Answer from the drawing. Dimensions are ordinates in mm from the lowest x, y and z of the part. Coordinates: 2 decimals unless noted, no trailing zeros. Loops run counter-clockwise (first coordinate to the right, second up) from the corner with the lowest first, then second, coordinate; pieces in that order, holes last. Notation, with made-up numbers: M 34,14 L 48,14 A22 ccw 48,53 Z; hole C -14,9 d11. An arc over 180 degrees is marked long. Answer as CSV lines item,"result". Start each with the question number.
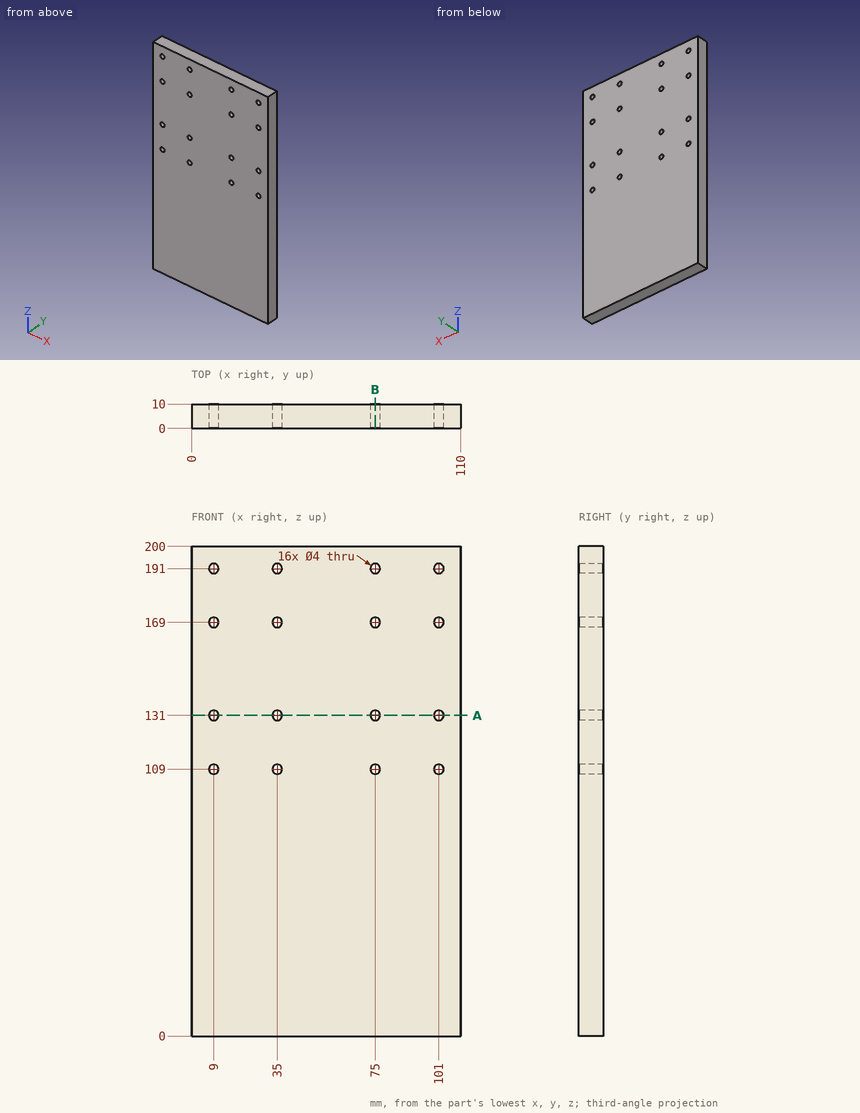
Item 1: Consider line 1 (Z direction, x = 75, y = 7.75); line 2 (X direction, y = 7.25, z = 169); line 3 (X direction, y = 8.25, z = 110.5). Determine where each line is inside the solid, lowest interval first.
Item 2: Section A-A on z = 131 is taken. Determine the outline of the cut face in (x, y).
Item 3: Section B-B on x = 75 is taken. Determine the outline of the cut face in (y, z).
Results are:
1,line 1,"0 to 107, 111 to 129, 133 to 167, 171 to 189, 193 to 200"
1,line 2,"0 to 7, 11 to 33, 37 to 73, 77 to 99, 103 to 110"
1,line 3,"0 to 7.68, 10.32 to 33.68, 36.32 to 73.68, 76.32 to 99.68, 102.32 to 110"
2,outline,"M 0,0 L 7,0 L 7,10 L 0,10 Z; M 11,0 L 33,0 L 33,10 L 11,10 Z; M 37,0 L 73,0 L 73,10 L 37,10 Z; M 77,0 L 99,0 L 99,10 L 77,10 Z; M 103,0 L 110,0 L 110,10 L 103,10 Z"
3,outline,"M 0,0 L 10,0 L 10,107 L 0,107 Z; M 0,111 L 10,111 L 10,129 L 0,129 Z; M 0,133 L 10,133 L 10,167 L 0,167 Z; M 0,171 L 10,171 L 10,189 L 0,189 Z; M 0,193 L 10,193 L 10,200 L 0,200 Z"
